Design review of the part built by this model. Coordinates are the model's own, in mm. A direction names the side the tool comes from. Coordinates: 2 decimals unless noted, no trailing zeros. Write each loop counter-clockwise with the first axis right and the second up, starting at its lowest first coordinate (ties: lowest second). Pieces come first, ordered by that corner, then holes.
Q1. Add section A-A, the plane x = 9. Give the boundary of the cut face in (y, z).
Q2. Add section B-B, the plane y = 44.5. Give the boundary of the cut face in (x, z).
Q3. Add section D-D, the plane y = 35.5. Give the boundary of the cut face in (x, z).
Q4. Machinability: for faces 4 (the face through (-21.21, 34.53, 0.25)), 5 (the face through (0, 41, 0.5)), which of the approach directions +Z, -Z, +X, -X, +Y, -Y give a long, thin tool a straight path to every point of the face, cutting with its end or side? Answer none if there is none.
Q5. The part is to be moulded in two halves that separate along X. For faces 1 (the face through (-9.543, 44.762, 0.246)), 2 (the face through (-0.4, 50, 0.2)), 3 (the face through (0, 41, 0)), say which applies: +X half, -X half, draft (parallel to the pull), parting line (faces both ways), or undercut.
Q6. Add section C-C, the plane z = 0.3. Give the boundary of the cut face in (x, y) (1 decimal).
Q7. To check wall thickness, follow probe 1 along X at (y, z) = (44, 0.2); probe 2 along Y at (x, z) = (7.5, 0.35); probe 3 along X at (y, z) = (44.5, 0.15). State the ranges of each line that lie inside material, in increasing order.
Autodesk Inventor part; units mm, degrees
ref_plane "YZ Plane" through (0, 0, 0) normal (1, 0, 0) x (0, 1, 0)
ref_plane "XZ Plane" through (0, 0, 0) normal (0, 1, 0) x (-1, 0, 0)
ref_plane "XY Plane" through (0, 0, 0) normal (0, 0, 1) x (1, 0, 0)
sketch "Sketch1" plane through (0, 0, 0) normal (0, 0, 1) x (1, 0, 0)
  circle A0 centre (-7.9561, 43.545) radius 2
  circle A1 centre (7.8751, 43.545) radius 2
  line L0 (-11.8358, 51) -> (11.6369, 51)
  line L1 (-11.8358, 49.5789) -> (-11.8358, 51)
  arc A2 (-11.8358, 49.5789) -> (-25.0147, 44.2928) centre (0, 1) ccw
  line L2 (-25.0147, 44.2928) -> (-26.0147, 44.2928)
  line L3 (-26.0147, 32.5428) -> (-26.0147, 44.2928)
  line L4 (-25.0147, 32.5428) -> (-26.0147, 32.5428)
  arc A3 (-17.1289, 36.2245) -> (-25.0147, 32.5428) centre (0, -10.75) ccw
  line L5 (17.1289, 36.2245) -> (-17.1289, 36.2245)
  arc A4 (25.0147, 32.5428) -> (17.1289, 36.2245) centre (0, -10.75) ccw
  line L6 (25.0147, 32.5428) -> (26.0147, 32.5428)
  line L7 (26.0147, 32.5428) -> (26.0147, 44.2928)
  line L8 (25.0147, 44.2928) -> (26.0147, 44.2928)
  arc A5 (25.0147, 44.2928) -> (11.6369, 49.627) centre (0, 1) ccw
  line L9 (11.6369, 49.627) -> (11.6369, 51)
  circle A6 centre (7.8751, 43.545) radius 2
  circle A7 centre (-7.9561, 43.545) radius 2
  arc A8 (26.0147, 42.6994) -> (-26.0147, 42.6994) centre (0, 0) ccw
  line L10 (-26.0147, 42.6994) -> (-26.0147, 32.5428)
  line L11 (-26.0147, 32.5428) -> (-25.0147, 32.5428)
  arc A9 (-17.1289, 36.2245) -> (-25.0147, 32.5428) centre (0, -10.75) ccw
  line L12 (-17.1289, 36.2245) -> (17.1289, 36.2245)
  arc A10 (25.0147, 32.5428) -> (17.1289, 36.2245) centre (0, -10.75) ccw
  line L13 (26.0147, 32.5428) -> (25.0147, 32.5428)
  line L14 (26.0147, 32.5428) -> (26.0147, 42.6994)
  point P0 (-26.0147, 42.6994)
  point P1 (-25.0147, 32.5428)
extrude "Extrusion1" add sketch "Sketch1" along normal blind 0.5 contours A8 L7 L6 A4 L5 A3 L4 L3
properties part number "warda"
Here are the results:
1. outline: (36.22, 0) - (41.89, 0) - (41.89, 0.5) - (36.22, 0.5) - close; (45.2, 0) - (49.18, 0) - (49.18, 0.5) - (45.2, 0.5) - close
2. outline: (-22.8, 0) - (-9.71, 0) - (-9.71, 0.5) - (-22.8, 0.5) - close; (-6.2, 0) - (6.12, 0) - (6.12, 0.5) - (-6.2, 0.5) - close; (9.63, 0) - (22.8, 0) - (22.8, 0.5) - (9.63, 0.5) - close
3. outline: (-26.01, 0) - (-19, 0) - (-19, 0.5) - (-26.01, 0.5) - close; (19, 0) - (26.01, 0) - (26.01, 0.5) - (19, 0.5) - close
4. face 4: +Z, -Z, -Y
4. face 5: +Z, +X, -X, +Y, -Y
5. face 1: undercut
5. face 2: parting line
5. face 3: draft
6. outline: (-26, 32.5) - (-25, 32.5) arc R50 cw to (-17.1, 36.2) - (17.1, 36.2) arc R50 cw to (25, 32.5) - (26, 32.5) - (26, 42.7) arc R50 ccw to (-26, 42.7) - close; hole circle Ø4 at (-8, 43.5); hole circle Ø4 at (7.9, 43.5)
7. probe 1: x = -23.75 to -9.9, -6.01 to 5.93, 9.82 to 23.75
7. probe 2: y = 36.22 to 41.58, 45.51 to 49.43
7. probe 3: x = -22.8 to -9.71, -6.2 to 6.12, 9.63 to 22.8
